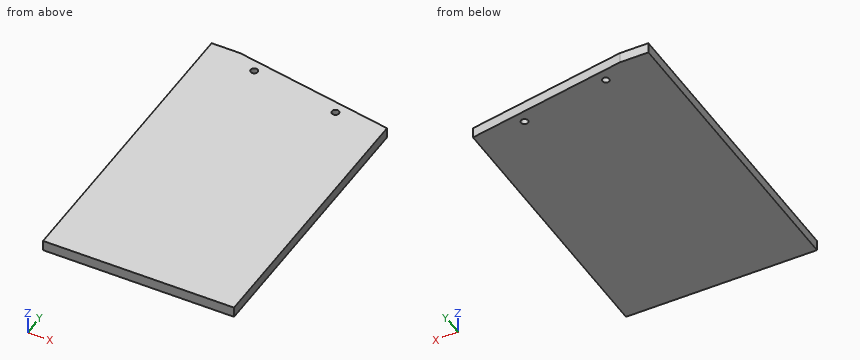
```python
from build123d import *

# Parameters (mm, degrees)
BOSS_EXTRUDE1_DEPTH            = 11.90625
F_5_16_0_3125_DIAMETER_HOLE1_D = 7.9375
SKETCH4_W                      = 220.489922176
SKETCH4_H                      = 247.65
CUT_EXTRUDE1_DEPTH             = 12.90625


with BuildPart() as part:
    # Sketch1 → Boss-Extrude1 (new body)
    with BuildSketch(Plane.XY):
        Polygon((151.023557582, 150.952887465), (-32.640904146, 183.337887465), (-64.876442418, 183.337887465), (-64.876442418, -413.562112535), (-32.640904146, -413.562112535), (151.023557582, -381.177112535), align=None)
    extrude(amount=BOSS_EXTRUDE1_DEPTH)

    # 5/16 (0.3125) Diameter Hole1 (through all)
    with Locations(Plane.XY.offset(11.90625)):
        with Locations((94.359095854, 148.048442944), (-7.240904146, 165.963264184), (-7.240904146, -396.187489254), (94.359095854, -378.272668014)):
            Hole(F_5_16_0_3125_DIAMETER_HOLE1_D / 2)

    # Sketch4 → Cut-Extrude1 (cut, through all)
    with BuildSketch(Plane(origin=(0, 0, 0), x_dir=(-1, 0, 0), z_dir=(0, 0, -1))):
        with Locations((-45.36851867, -289.737112535)):
            Rectangle(SKETCH4_W, SKETCH4_H)
    extrude(amount=-CUT_EXTRUDE1_DEPTH, mode=Mode.SUBTRACT)


solid = part.part
```
Can you work these out from the model? Positions are in its coordinate system, mm. Give positions to 0.01 mm unless a question says otherwise; leave off trailing zeros. Order: outer loops, then holes, each group sorted by start corner. A loop starts at its lowest first (then second) coordinate and runs counter-clockwise, first axis right, second up. Notation, with made-up numbers: (-2, -26) - (25, -26) arc R11 ccw to (25, -13) - close; hole circle Ø5 at (-19.5, -38.75). An arc over 180 degrees is marked (long way). Use a Markdown table: item, result. Add a question column.
Q1. If we section it at B-B on x = 54.5: Write out the boundary of the cut face in (y, z).
Q2. If we section it at A-A on z = 5: Write out the boundary of the cut face in (x, y).
Q3. Please list where these lines run through material, in increasing order: line 1 along Y through (x, z) = (25, 7); line 2 along Y through (x, z) = (105.5, 5).
Q4. If we section it at C-C on x = 119: Write out the boundary of the cut face in (y, z), plus the area to 3 significant figures.
Answers follow:
| question | item | result |
|---|---|---|
| 1 | outline | (-165.91, 0) - (167.97, 0) - (167.97, 11.91) - (-165.91, 11.91) - close |
| 2 | outline | (-64.88, -165.91) - (151.02, -165.91) - (151.02, 150.95) - (-32.64, 183.34) - (-64.88, 183.34) - close; hole circle Ø7.94 at (-7.24, 165.96); hole circle Ø7.94 at (94.36, 148.05) |
| 3 | line 1 | y = -165.91 to 173.17 |
| 3 | line 2 | y = -165.91 to 158.98 |
| 4 | outline | (-165.91, 0) - (156.6, 0) - (156.6, 11.91) - (-165.91, 11.91) - close |
| 4 | area | 3,840 mm^2 |
